from build123d import *

# Parameters (mm, degrees)
SKETCH_R        = 1.7
PAD_DEPTH       = 13
SKETCH001_W     = 83
SKETCH001_H     = 103
POCKET_DEPTH    = 10
SKETCH002_W     = 18
SKETCH002_H     = 8.6
POCKET001_DEPTH = 11
SKETCH004_R     = 3
POCKET002_DEPTH = 3.1
SKETCH006_R     = 3
POCKET003_DEPTH = 3.1
SKETCH007_R     = 3
POCKET004_DEPTH = 3.1
SKETCH005_R     = 3
POCKET005_DEPTH = 3.1


with BuildPart() as part:
    # Sketch → Pad (new body)
    with BuildSketch(Plane.XY):
        with BuildLine():
            ThreePointArc((-45.25, 60), (-48.785534, 58.535534), (-50.25, 55))
            Line((-50.25, -55), (-50.25, 55))
            ThreePointArc((-50.25, -55), (-48.785534, -58.535534), (-45.25, -60))
            Line((45.25, -60), (-45.25, -60))
            ThreePointArc((45.25, -60), (48.785534, -58.535534), (50.25, -55))
            Line((50.25, 55), (50.25, -55))
            ThreePointArc((50.25, 55), (48.785534, 58.535534), (45.25, 60))
            Line((-45.25, 60), (45.25, 60))
        make_face()
        with Locations((-45.25, 55)):
            Circle(SKETCH_R, mode=Mode.SUBTRACT)
        with Locations((45.25, 55)):
            Circle(SKETCH_R, mode=Mode.SUBTRACT)
        with Locations((45.25, -55)):
            Circle(SKETCH_R, mode=Mode.SUBTRACT)
        with Locations((-45.25, -55)):
            Circle(SKETCH_R, mode=Mode.SUBTRACT)
    extrude(amount=PAD_DEPTH)

    # Sketch001 (on Face14 of Pad) → Pocket (cut)
    with BuildSketch(Plane.XY.offset(13)):
        Rectangle(SKETCH001_W, SKETCH001_H)
    extrude(amount=-POCKET_DEPTH, mode=Mode.SUBTRACT)

    # Sketch002 (on Face2 of Pocket) → Pocket001 (cut)
    with BuildSketch(Plane(origin=(0, 60, 0), x_dir=(-1, 0, 0), z_dir=(0, 1, 0))):
        with Locations((-23.25, 7.3)):
            Rectangle(SKETCH002_W, SKETCH002_H)
    extrude(amount=-POCKET001_DEPTH, mode=Mode.SUBTRACT)

    # Sketch004 (on Face4 of Pocket001) → Pocket002 (cut)
    with BuildSketch(Plane(origin=(0, 0, 0), x_dir=(1, 0, 0), z_dir=(0, 0, -1))):
        with Locations((-45.25, -55)):
            Circle(SKETCH004_R)
    extrude(amount=-POCKET002_DEPTH, mode=Mode.SUBTRACT)

    # Sketch006 (on Face4 of Pocket001) → Pocket003 (cut)
    with BuildSketch(Plane(origin=(0, 0, 0), x_dir=(1, 0, 0), z_dir=(0, 0, -1))):
        with Locations((-45.25, 55)):
            Circle(SKETCH006_R)
    extrude(amount=-POCKET003_DEPTH, mode=Mode.SUBTRACT)

    # Sketch007 (on Face4 of Pocket001) → Pocket004 (cut)
    with BuildSketch(Plane(origin=(0, 0, 0), x_dir=(1, 0, 0), z_dir=(0, 0, -1))):
        with Locations((45.25, 55)):
            Circle(SKETCH007_R)
    extrude(amount=-POCKET004_DEPTH, mode=Mode.SUBTRACT)

    # Sketch005 (on Face4 of Pocket001) → Pocket005 (cut)
    with BuildSketch(Plane(origin=(0, 0, 0), x_dir=(1, 0, 0), z_dir=(0, 0, -1))):
        with Locations((45.25, -55)):
            Circle(SKETCH005_R)
    extrude(amount=-POCKET005_DEPTH, mode=Mode.SUBTRACT)


solid = part.part
Check sheet for the modelled part. Datum: model origin and axes. Units: mm. A direction names the side the tool comes from. Give positions to 0.01 mm unless a question says otherwise; leave off trailing zeros. Order: outer loops, then holes, each group sorted by start corner. A loop starts at its lowest first (then second) coordinate and runs counter-clockwise, first axis right, second up. Notation, with made-up numbers: (51, 31.25) - (99, 31.25) arc R18 ccw to (99, 53.25) - close; hole circle Ø5 at (-37.5, 32.5). An arc over 180 degrees is marked (long way). Answer as CSV lines item,"result".
1. Section check A-A (z = 4.75). Record the boundary of the cut face in (x, y), then the cut area to 3 significant figures.
Result sheet:
outline,"(-50.25, -55) arc R5 ccw to (-45.25, -60) - (45.25, -60) arc R5 ccw to (50.25, -55) - (50.25, 55) arc R5 ccw to (45.25, 60) - (32.25, 60) - (32.25, 51.5) - (41.5, 51.5) - (41.5, -51.5) - (-41.5, -51.5) - (-41.5, 51.5) - (14.25, 51.5) - (14.25, 60) - (-45.25, 60) arc R5 ccw to (-50.25, 55) - close; hole circle Ø3.4 at (-45.25, -55); hole circle Ø3.4 at (-45.25, 55); hole circle Ø3.4 at (45.25, -55); hole circle Ø3.4 at (45.25, 55)"
area,"3,300 mm²"
2. Scan lines: probe 1 along X at (y, z) = (55, 7.75); probe 2 along X at (y, z) = (-55, 1); probe 3 along Y at (x, z) = (45.25, 7). Record each from-to range of solid material in increasing order. Write a range as from..to.
Result sheet:
probe 1,"-50.25..-46.95, -43.55..14.25, 32.25..43.55, 46.95..50.25"
probe 2,"-50.25..-48.25, -42.25..42.25, 48.25..50.25"
probe 3,"-60..-56.7, -53.3..53.3, 56.7..60"
3. Go/stop test with flat-tipped pins: P1, Ø1, axis at x = 13, y = 34.5, coming from the +Z side; P2, Ø5.5, axis at x = -45.25, y = -55, coming from the -Z side. Record where each tip stops, or that it passes through.
Result sheet:
P1,"z = 3"
P2,"z = 3.1"
4. Section check C-C (y = -13). Record the boundary of the cut face in (x, z), then the cut area to 4 significant figures.
Result sheet:
outline,"(-50.25, 0) - (50.25, 0) - (50.25, 13) - (41.5, 13) - (41.5, 3) - (-41.5, 3) - (-41.5, 13) - (-50.25, 13) - close"
area,"476.5 mm²"
5. Tool access check on faces 4 (the face through (1, -60, 6)), 5 (the face through (41.5, -1, 8)), 6 (the face through (-45, 57, 3.1)), 7 (the face through (32.25, 56, 7)). Record the directions out of +Z, -Z, +X, -X, +Y, -Y that give a thin tool (end or side, any length) a straight path to the whole face; none if there is none.
Result sheet:
face 4,"+Z, -Z, +X, -X, -Y"
face 5,"+Z"
face 6,"-Z"
face 7,"+Y"
6. Mould release check, pull along Z, two halves, no side actions. Record for faces 1 (the face through (47, -54, 3.1)), 2 (the face through (-45, 1, 13)), 3 (the face through (23, 56, 11.6)): released by +Z, released by -Z, zero draft, split by the parting line, or undercut.
Result sheet:
face 1,"released by -Z"
face 2,"released by +Z"
face 3,"undercut"
7. Section check B-B (x = 3). Record the boundary of the cut face in (y, z), then the cut area to 3 significant figures.
Result sheet:
outline,"(-60, 0) - (60, 0) - (60, 13) - (51.5, 13) - (51.5, 3) - (-51.5, 3) - (-51.5, 13) - (-60, 13) - close"
area,"530 mm²"
